Here's how the part is built. I have some questions about the finished solid (model axes, mm). A direction names the side the tool comes from. Coordinates: 2 decimals unless noted, no trailing zeros. Write each loop counter-clockwise with the first axis right and the second up, starting at its lowest first coordinate (ties: lowest second). Pieces come first, ordered by that corner, then holes.
```python
from build123d import *

# Parameters (mm, degrees)
SKETCH1_R                                      = 16.891
BOSS_EXTRUDE1_DEPTH                            = 43.3324
SKETCH9_R                                      = 9.525
CUT_EXTRUDE6_DEPTH                             = 50.480386536
SKETCH10_R                                     = 11.43
BOSS_EXTRUDE2_DEPTH                            = 19.05
CUT_EXTRUDE7_START                             = -39.36365
SKETCH11_R                                     = 9.525
CUT_EXTRUDE7_DEPTH                             = 39.36365
CUT_EXTRUDE8_START                             = -3.96875
CUT_EXTRUDE8_DEPTH                             = 3.96875
CSK_FOR_2_FLAT_HEAD_MACHINE_SCREW1_D           = 2.2606
CSK_FOR_2_FLAT_HEAD_MACHINE_SCREW1_CSINK_D     = 4.3688
CSK_FOR_2_FLAT_HEAD_MACHINE_SCREW1_CSINK_ANGLE = 82
CIRPATTERN1_COUNT                              = 6
F_1_2_0_4_DIAMETER_HOLE1_D                     = 10.16
F_1_2_0_4_DIAMETER_HOLE1_DEPTH                 = 12.7
F_1_2_0_4_DIAMETER_HOLE1_TIP                   = 3.052371945
FILLET1_R                                      = 1.27
SKETCH16_W                                     = 16.51
SKETCH16_H                                     = 16.51
CUT_EXTRUDE9_DEPTH                             = 12.7


with BuildPart() as part:
    # Sketch1 → Boss-Extrude1 (new body)
    with BuildSketch(Plane.XY):
        Circle(SKETCH1_R)
    extrude(amount=BOSS_EXTRUDE1_DEPTH)

    # Sketch9 → Cut-Extrude6 (cut, through all)
    with BuildSketch(Plane(origin=(0, 0, 0), x_dir=(-1, 0, 0), z_dir=(0, 0, -1))):
        Circle(SKETCH9_R)
        with BuildLine():
            ThreePointArc((-5.359640753, -7.874), (0, -9.525), (5.359640753, -7.874))
            Line((5.359640753, -7.874), (-5.359640753, -7.874))
        make_face()
        with BuildLine():
            ThreePointArc((-7.874, 5.359640753), (-9.525, 0), (-7.874, -5.359640753))
            Line((-7.874, -5.359640753), (-7.874, 5.359640753))
        make_face()
        with BuildLine():
            Line((-5.359640753, 7.874), (5.359640753, 7.874))
            ThreePointArc((5.359640753, 7.874), (0, 9.525), (-5.359640753, 7.874))
        make_face()
        with BuildLine():
            Line((7.874, 5.359640753), (7.874, -5.359640753))
            ThreePointArc((7.874, -5.359640753), (9.102897204, -2.804084075), (9.525, 0))
            ThreePointArc((9.525, 0), (9.102897204, 2.804084075), (7.874, 5.359640753))
        make_face()
    extrude(amount=-CUT_EXTRUDE6_DEPTH, mode=Mode.SUBTRACT)

    # Sketch10 → Boss-Extrude2 (add)
    # profile 1 of 2: a face of its own
    with BuildSketch(Plane(origin=(0, 0, 0), x_dir=(-1, 0, 0), z_dir=(0, 0, -1))):
        Circle(SKETCH10_R)
        with BuildLine():
            ThreePointArc((-5.359640753, -7.874), (-4.453933477, 8.419507206), (9.525, 0))
            ThreePointArc((9.525, 0), (8.419507206, -4.453933477), (5.359640753, -7.874))
            ThreePointArc((5.359640753, -7.874), (0, -9.525), (-5.359640753, -7.874))
        make_face(mode=Mode.SUBTRACT)
    # profile 2 of 2: a face of its own
    with BuildSketch(Plane(origin=(0, 0, 0), x_dir=(-1, 0, 0), z_dir=(0, 0, -1))):
        Circle(SKETCH10_R)
        with BuildLine():
            ThreePointArc((-5.359640753, -7.874), (-4.453933477, 8.419507206), (9.525, 0))
            ThreePointArc((9.525, 0), (8.419507206, -4.453933477), (5.359640753, -7.874))
            ThreePointArc((5.359640753, -7.874), (0, -9.525), (-5.359640753, -7.874))
        make_face(mode=Mode.SUBTRACT)
    extrude(amount=-BOSS_EXTRUDE2_DEPTH)

    # Sketch11 → Cut-Extrude7 (cut)
    with BuildSketch(Plane.XY.offset(43.3324).offset(CUT_EXTRUDE7_START)):
        with BuildLine():
            Line((-9.153468369, -2.634319991), (-10.984162043, -3.161183989))
            ThreePointArc((-10.984162043, -3.161183989), (1.596234295, -11.317991698), (11.43, 0))
            ThreePointArc((11.43, 0), (1.610471515, 11.315974615), (-10.976173491, 3.188810986))
            Line((-10.976173491, 3.188810986), (-9.146811242, 2.657342489))
            ThreePointArc((-9.146811242, 2.657342489), (1.342059596, 9.429978846), (9.525, 0))
            ThreePointArc((9.525, 0), (1.330195246, -9.431659748), (-9.153468369, -2.634319991))
        make_face()
        with Locations(Location((0, 0, 0), (0, 0, 180))):
            Circle(SKETCH11_R)
        with BuildLine():
            ThreePointArc((-10.984162043, -3.161183989), (-11.297244321, 0.014212394), (-10.976173491, 3.188810986))
            Line((-10.976173491, 3.188810986), (0, 0))
            Line((0, 0), (-10.984162043, -3.161183989))
        make_face()
        with BuildLine():
            ThreePointArc((-10.976173491, 3.188810986), (-11.429990955, 0.014379395), (-10.984162043, -3.161183989))
            ThreePointArc((-10.984162043, -3.161183989), (-11.297244321, 0.014212394), (-10.976173491, 3.188810986))
        make_face()
    extrude(amount=CUT_EXTRUDE7_DEPTH, mode=Mode.SUBTRACT)

    # Sketch11<4> → Cut-Extrude8 (cut)
    with BuildSketch(Plane.XY.offset(43.3324).offset(CUT_EXTRUDE8_START)):
        with BuildLine():
            ThreePointArc((-10.976173491, 3.188810986), (-11.297244321, 0.014212394), (-10.984162043, -3.161183989))
            Line((-10.984162043, -3.161183989), (0, 0))
            Line((0, 0), (-10.976173491, 3.188810986))
        make_face()
        with BuildLine():
            ThreePointArc((-10.976173491, 3.188810986), (-11.429990955, 0.014379395), (-10.984162043, -3.161183989))
            ThreePointArc((-10.984162043, -3.161183989), (-11.297244321, 0.014212394), (-10.976173491, 3.188810986))
        make_face()
        with BuildLine():
            Line((-16.232150575, -4.67152745), (-10.984162043, -3.161183989))
            ThreePointArc((-10.984162043, -3.161183989), (-11.429990955, 0.014379395), (-10.976173491, 3.188810986))
            Line((-10.976173491, 3.188810986), (-16.220345269, 4.712354013))
            ThreePointArc((-16.220345269, 4.712354013), (-16.925737574, 0.021293268), (-16.232150575, -4.67152745))
        make_face()
        with BuildLine():
            Line((0, 0), (-10.984162043, -3.161183989))
            ThreePointArc((-10.984162043, -3.161183989), (1.596234295, -11.317991698), (11.43, 0))
            ThreePointArc((11.43, 0), (1.610471515, 11.315974615), (-10.976173491, 3.188810986))
            Line((-10.976173491, 3.188810986), (0, 0))
        make_face()
    cut_extrude8 = extrude(amount=CUT_EXTRUDE8_DEPTH, mode=Mode.SUBTRACT)

    # CSK for #2 Flat Head Machine Screw1 (through all)
    with Locations(Plane(origin=(0, 0, 0), x_dir=(-1, 0, 0), z_dir=(0, 0, -1))):
        with Locations((11.671937945, 6.75838911)):
            csk_for_2_flat_head_machine_screw1 = CounterSinkHole(CSK_FOR_2_FLAT_HEAD_MACHINE_SCREW1_D / 2, CSK_FOR_2_FLAT_HEAD_MACHINE_SCREW1_CSINK_D / 2, counter_sink_angle=CSK_FOR_2_FLAT_HEAD_MACHINE_SCREW1_CSINK_ANGLE)

    # CirPattern1: Cut-Extrude8, CSK for #2 Flat Head Machine Screw1 ×6 about axis
    cirpattern1_axis = Axis((0, 0, 0), (0, 0, 1))
    add([cut_extrude8.rotate(cirpattern1_axis, i * 360 / CIRPATTERN1_COUNT) for i in range(1, CIRPATTERN1_COUNT)], mode=Mode.SUBTRACT)
    add([csk_for_2_flat_head_machine_screw1.rotate(cirpattern1_axis, i * 360 / CIRPATTERN1_COUNT) for i in range(1, CIRPATTERN1_COUNT)], mode=Mode.SUBTRACT)

    # 1/2 (0.4) Diameter Hole1
    with Locations(Plane(origin=(16.890986634, -0.02124955, 14.908061188), x_dir=(0.001258039772, 0.999999208668, 0), z_dir=(0.999999208668, -0.001258039772, 0))):
        with Locations((0, 0)):
            Hole(F_1_2_0_4_DIAMETER_HOLE1_D / 2, depth=F_1_2_0_4_DIAMETER_HOLE1_DEPTH)
            with Locations((0, 0, -(F_1_2_0_4_DIAMETER_HOLE1_DEPTH + F_1_2_0_4_DIAMETER_HOLE1_TIP / 2))):  # 118° drill point
                Cone(0, F_1_2_0_4_DIAMETER_HOLE1_D / 2, F_1_2_0_4_DIAMETER_HOLE1_TIP, mode=Mode.SUBTRACT)

    # Fillet1
    # the kernel refuses this fillet: 1.27 mm, written as the material it takes off along each edge
    with BuildSketch(Plane(origin=(0, 0, 0), x_dir=(1, 0, 0), z_dir=(0, -1, 0))) as fillet1_piece_1:
        with BuildLine():
            CenterArc((16.891 - FILLET1_R, FILLET1_R), FILLET1_R, 270, 90)
            Line((16.891 - FILLET1_R, 0), (16.891, 0))
            Line((16.891, 0), (16.891, FILLET1_R))
        make_face()
    revolve(axis=Axis((0, 0, 0), (0, 0, 1)), mode=Mode.SUBTRACT)

    # Sketch16 → Cut-Extrude9 (cut)
    with BuildSketch(Plane(origin=(0, 0, 0), x_dir=(-1, 0, 0), z_dir=(0, 0, -1))):
        with Locations((0.016967686, 0.019651839)):
            Rectangle(SKETCH16_W, SKETCH16_H)
    extrude(amount=-CUT_EXTRUDE9_DEPTH, mode=Mode.SUBTRACT)


solid = part.part
```
1) On a 3-axis mill with a long thin cutter (end or side, diameter ignored), from which of +Z, -Z, +X, -X, +Y, -Y can I reach the whole of each face in a straight line? I mean faces 1 (the face through (0, -10, 3.969)), 2 (the face through (10.19, 9.77, 41.32)), 3 (the face through (-8.272, -7, 3)), 4 (the face through (13.645, 3.927, 41.32)). Say none if no direction works.
Values follow:
face 1: +Z
face 2: +Z, +Y
face 3: -Z
face 4: +Z, +X
2) Imagine slicing it at A-A on z = 40. Count the separate pieces of the cut face and the enclosed holes in it, then the cut area to 3 significant figures.
Values follow:
separate pieces: 6
enclosed holes: 6
area: 201 mm2
3) Will these pins go through, and if not, where does the flat tip stop? pin 1 (1.6 mm diameter, centred on x = 10, y = 2.5, fed in from +Z); pin 2 (1.8 mm diameter, centred on y = 6, z = 4.5, fed in from +X); pin 3 (2.5 mm diameter, centred on x = 7, y = 13.5, fed in from +Z).
Values follow:
pin 1: stops at z = 3.97
pin 2: stops at x = 16.1
pin 3: stops at z = 39.36
4) Imagine slicing it at B-B on z = 34. Please give me the cut outline in (x, y), then the cut area to 3 significant figures.
Values follow:
outline: circle Ø33.78 at (0, 0); hole circle Ø2.26 at (-11.69, -6.73); hole circle Ø2.26 at (-11.67, 6.76); hole circle Ø22.86 at (0, 0); hole circle Ø2.26 at (-0.02, -13.49); hole circle Ø2.26 at (0.02, 13.49); hole circle Ø2.26 at (11.67, -6.76); hole circle Ø2.26 at (11.69, 6.73)
area: 462 mm2
5) I need wall thicknesses on probe 1 along Y at (x, z) = (0, 27.5); probe 2 along X at (y, z) = (-11.5, 40.5); probe 3 along X at (y, z) = (7, 22.5). Which ranges of each line are inside material? Lowest first, please.
Values follow:
probe 1: y = -16.89 to -14.62, -12.36 to -11.43, 11.43 to 12.36, 14.62 to 16.89
probe 2: x = -12.37 to -11.99, -2.86 to 2.82, 11.93 to 12.37
probe 3: x = -15.37 to -12.78, -10.57 to -9.04, 9.04 to 10.59, 12.79 to 15.37
6) We'd pull the mould along Y, two halves only. Please class faces 5 (the face through (0, 15, 43.332)), 6 (the face through (-3.369, 13.715, 41.32)), 7 (the face through (-10.19, -9.77, 41.32)), 8 (the face through (-10.22, 9.85, 41.32)): pulls with the +Y half, pulls with the -Y half, needs draft (parallel to the pull), parting line crosses it, or undercut.
Values follow:
face 5: needs draft
face 6: undercut
face 7: pulls with the -Y half
face 8: pulls with the +Y half
7) Imagine slicing it at C-C on z = 8.5. Please give me the cut outline in (x, y), then the cut area to 3 significant figures.
Values follow:
outline: circle Ø33.78 at (0, 0); hole circle Ø2.26 at (-11.69, -6.73); hole circle Ø2.26 at (-11.67, 6.76); hole (-8.27, -8.24) - (-7.93, -8.24) arc R11.43 ccw to (7.93, -8.24) - (8.24, -8.24) - (8.24, -7.92) arc R11.43 ccw to (8.24, 7.92) - (8.24, 8.27) - (7.89, 8.27) arc R11.43 ccw to (-7.89, 8.27) - (-8.27, 8.27) - (-8.27, 7.89) arc R11.43 ccw to (-8.27, -7.89) - close; hole circle Ø2.26 at (-0.02, -13.49); hole circle Ø2.26 at (0.02, 13.49); hole circle Ø2.26 at (11.67, -6.76); hole circle Ø2.26 at (11.69, 6.73)
area: 462 mm2
